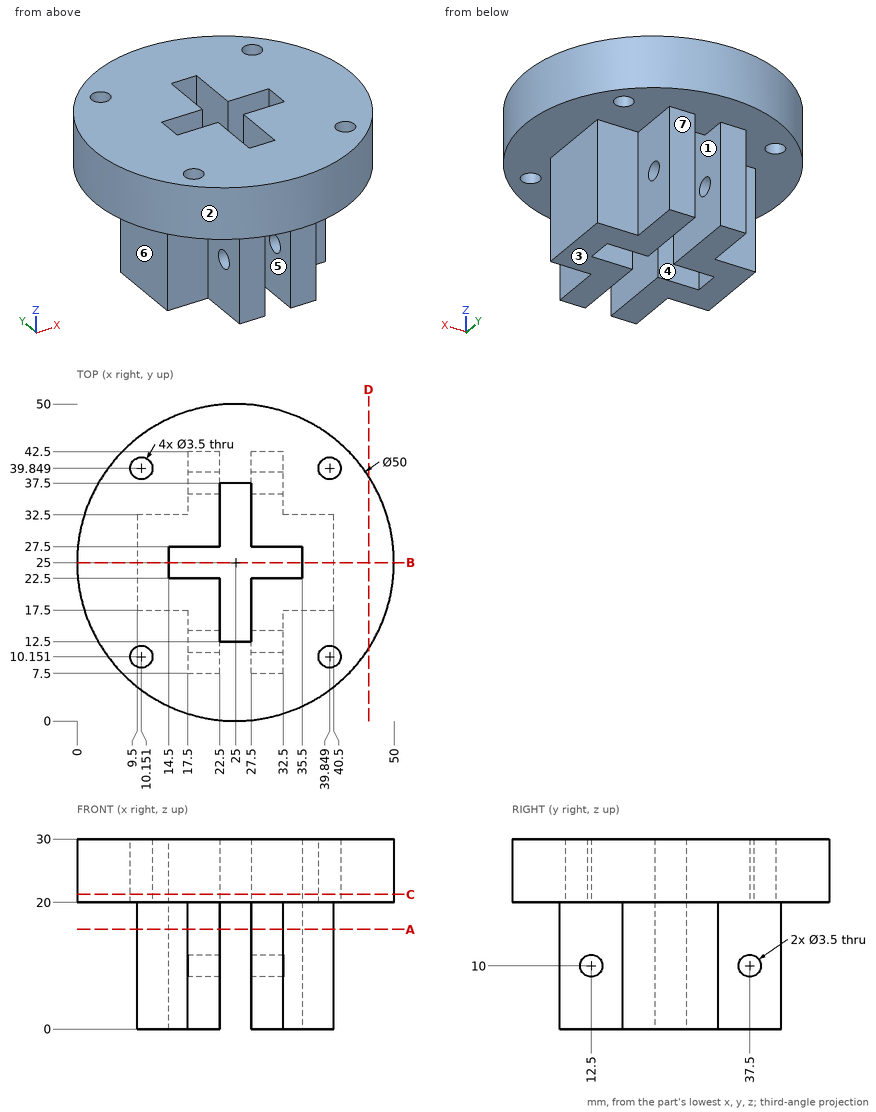
Check sheet for the drawn part. Datum: minimum x, y, z corner. Units: mm. A direction names the side the tool comes from. Give positions to 0.01 mm unless a question says otherwise; leave off trailing zeros. Write each loop counter-clockwise with the first axis right and the second up, starting at its lowest first coordinate (ties: lowest second). Pieces come first, ordered by that corner, then holes.
(1) Cross-section at D-D (x = 46). Enter the section's corners in (y, z) (1 decimal), plus the area to 3 significant figures.
(2) Cross-section at B-B (y = 25). Enter the section's corners in (x, z).
(3) Material ranges on line 1 (Y direction, x = 31.1, z = 10); line 2 (X direction, y = 13.5, z = 14); line 3 (Y direction, x = 20, z = 16.25), recorded low to high.
(4) Access from +Z, -Z, +X, -X, +Y, -Y to the whole of each face (thin tool, end or side, straight path). Record for the marked faces 4, 5, 6 and 7.
(5) Cross-section at C-C (z = 21.25). Enter the section's corners in (x, y).
(6) Cross-section at A-A (z = 15.75). Enter the section's corners in (x, y), plus the area to 3 significant figures.
(7) Mould release check, pull along X, two halves, no side actions. Record for the marked faces 1, 2 and 3: +X half, -X half, draft (parallel to the pull), parting line (faces both ways), or undercut.
(8) Gauge pin test, flat ends, axial feed: pin 1 (4 mm diameter, centred on x = 25, z = 22.5, fed in from +Y); pin 2 (4.5 mm diameter, centred on y = 37.5, z = 10, fed in from +X); pin 3 (9 mm diameter, centred on x = 19.5, z = 19, fed in from -Y) (1 decimal). Record the tip position at first contact, or that the pin passes through.
Worked out:
1. outline: (11.4, 20) - (38.6, 20) - (38.6, 30) - (11.4, 30) - close
1. area: 271 mm2
2. outline: (0, 20) - (9.5, 20) - (9.5, 0) - (14.5, 0) - (14.5, 30) - (0, 30) - close; (35.5, 0) - (40.5, 0) - (40.5, 20) - (50, 20) - (50, 30) - (35.5, 30) - close
3. line 1: y = 7.5 to 10.75, 14.25 to 22.5, 27.5 to 35.75, 39.25 to 42.5
3. line 2: x = 17.5 to 22.5, 27.5 to 32.5
3. line 3: y = 7.5 to 22.5, 27.5 to 42.5
4. face 4: +Z, -Z
4. face 5: -Z
4. face 6: -Z, -X, +Y, -Y
4. face 7: -Z, +X, -X, +Y
5. outline: circle Ø50 at (25, 25); hole circle Ø3.5 at (10.15, 10.15); hole circle Ø3.5 at (10.15, 39.85); hole (14.5, 22.5) - (22.5, 22.5) - (22.5, 12.5) - (27.5, 12.5) - (27.5, 22.5) - (35.5, 22.5) - (35.5, 27.5) - (27.5, 27.5) - (27.5, 37.5) - (22.5, 37.5) - (22.5, 27.5) - (14.5, 27.5) - close; hole circle Ø3.5 at (39.85, 10.15); hole circle Ø3.5 at (39.85, 39.85)
6. outline: (9.5, 17.5) - (17.5, 17.5) - (17.5, 7.5) - (22.5, 7.5) - (22.5, 22.5) - (14.5, 22.5) - (14.5, 27.5) - (22.5, 27.5) - (22.5, 42.5) - (17.5, 42.5) - (17.5, 32.5) - (9.5, 32.5) - close; (27.5, 7.5) - (32.5, 7.5) - (32.5, 17.5) - (40.5, 17.5) - (40.5, 32.5) - (32.5, 32.5) - (32.5, 42.5) - (27.5, 42.5) - (27.5, 27.5) - (35.5, 27.5) - (35.5, 22.5) - (27.5, 22.5) - close
6. area: 510 mm2
7. face 1: undercut
7. face 2: parting line
7. face 3: draft
8. pin 1: stops at y = 50
8. pin 2: stops at x = 32.5
8. pin 3: stops at y = 0
